```python
from build123d import *

# Parameters (mm, degrees)
FASE1_SIZE                           = 0.5
FASE2_SIZE                           = 1.3
SCHNITT_LINEAR_AUSTRAGEN1_DEPTH      = 15.75
SCHNITT_LINEAR_AUSTRAGEN1_DEPTH_BACK = 15.75
SKIZZE4_OUTSIDE_W                    = 40.932
SKIZZE4_OUTSIDE_H                    = 40.932
SKIZZE4_OUTSIDE_W_2                  = 20
SKIZZE4_OUTSIDE_H_2                  = 17
SCHNITT_LINEAR_AUSTRAGEN2_DEPTH      = 0.5


with BuildPart() as part:
    # Skizze2 → Rotation1 (revolve)
    with BuildSketch(Plane(origin=(0, 0, 0), x_dir=(0, 0, -1), z_dir=(1, 0, 0))):
        Polygon((0, 14.75), (-1.5, 14.75), (-1.5, 13), (-2, 13), (-2, 5.942548531), (-2.8, 5.942548531), (-2.8, 5), (-16.75, 5), (-16.75, 3.125), (-2.65, 3.125), (-2.65, 0.9), (5.25, 0.9), (5.25, 2.5), (0, 2.5), (0, 7.5), (0.5, 7.5), (0.5, 9.5), (0, 9.5), (0, 12.65), (-0.8, 12.65), (-0.8, 14.15), (0, 14.15), align=None)
    revolve(axis=Axis((0, 0, -10.606367747), (0, 0, 1)))

    # Fase1
    fase1_edges = [part.edges().sort_by_distance(p)[0] for p in [
        (0, -14.75, 1.5),
    ]]
    chamfer(fase1_edges, length=FASE1_SIZE)

    # Fase2
    fase2_edges = [part.edges().sort_by_distance(p)[0] for p in [
        (0, -3.125, 16.75),
    ]]
    chamfer(fase2_edges, length=FASE2_SIZE)

    # Skizze3 → Schnitt-Linear austragen1 (cut, two sides)
    with BuildSketch(Plane(origin=(0, 0, 0), x_dir=(1, 0, 0), z_dir=(0, 1, 0))) as schnitt_linear_austragen1_sk:
        with BuildLine():
            Line((1.85, -8.6), (1.85, -16.75))
            ThreePointArc((1.85, -16.75), (0, -18.6), (-1.85, -16.75))
            Line((-1.85, -16.75), (-1.85, -8.6))
            ThreePointArc((-1.85, -8.6), (0, -6.75), (1.85, -8.6))
        make_face()
    extrude(amount=SCHNITT_LINEAR_AUSTRAGEN1_DEPTH, mode=Mode.SUBTRACT)
    extrude(schnitt_linear_austragen1_sk.sketch, amount=-SCHNITT_LINEAR_AUSTRAGEN1_DEPTH_BACK, mode=Mode.SUBTRACT)

    # Skizze4 outside → Schnitt-Linear austragen2 (cut)
    with BuildSketch(Plane(origin=(0, 0, -0.5), x_dir=(-1, 0, 0), z_dir=(0, 0, -1))):
        Rectangle(SKIZZE4_OUTSIDE_W, SKIZZE4_OUTSIDE_H)
        Rectangle(SKIZZE4_OUTSIDE_W_2, SKIZZE4_OUTSIDE_H_2, mode=Mode.SUBTRACT)
    extrude(amount=-SCHNITT_LINEAR_AUSTRAGEN2_DEPTH, mode=Mode.SUBTRACT)


solid = part.part
```
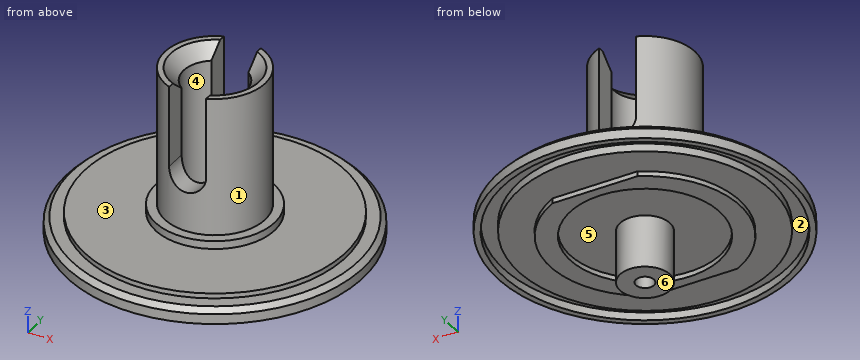
The model under review builds one solid part; all positions refer to its coordinate system, in mm. Face numbers are marked on the shaded views. A direction names the side the tool comes from. Coordinates: 2 decimals unless noted, no trailing zeros. Write each loop counter-clockwise with the first axis right and the second up, starting at its lowest first coordinate (ties: lowest second). Pieces come first, ordered by that corner, then holes.
1) The part is to be moulded in two halves that separate along Y. For the marked faces 1, 2 and 3, say which applies: pulls with the +Y half, pulls with the -Y half, needs draft (parallel to the pull), parting line crosses it, or undercut.
2) To check wall thickness, follow probe 1 along X at (y, z) = (0, 0.2); probe 2 along Y at (x, z) = (0, -0.1). State the ranges of each line that lie inside material, in increasing order.
3) Clearance check with flat-ended pins moving along their axes: pin 1 Ø1 at (x, y) = (9, 7.5) entering from +Z; pin 2 Ø2.5 at (y, z) = (4, 13) entering from +X; pin 3 Ø5 at (x, y) = (-1, -1) entering from +Z. State where each tip first meets the part, or that it passes through.
4) We need section A-A on z = 10.25. State the section outline as (x, y) points (3 decimals), then the cut area to 3 significant figures.
5) Machinability: for the marked faces 4, 5 and 6, which of the approach directions +Z, -Z, +X, -X, +Y, -Y give a long, thin tool a straight path to every point of the face, cutting with its end or side? Answer none if there is none.
6) We need section B-B on z = 4.5. State the section outline as (x, y) points (3 decimals), then the cut area to 3 significant figures.
Answer list:
1. face 1: parting line crosses it
1. face 2: undercut
1. face 3: needs draft
2. probe 1: x = -14.75 to -14.15, -12.65 to -0.9, 0.9 to 12.65, 14.15 to 14.75
2. probe 2: y = -8.5 to -7.5, -2.5 to -0.9, 0.9 to 2.5, 7.5 to 8.5
3. pin 1: stops at z = 2
3. pin 2: stops at x = 4.18
3. pin 3: stops at z = 16.24
4. outline: (-1.85, -4.645) - (-1.85, -2.519) arc R3.125 cw to (-1.85, 2.519) - (-1.85, 4.645) arc R5 ccw to start; (1.85, -4.645) arc R5 ccw to (1.85, 4.645) - (1.85, 2.519) arc R3.125 cw to (1.85, -2.519) - close
4. area: 33.4 mm2
5. face 4: +Z
5. face 5: -Z
5. face 6: -Z, +X, -X, +Y, -Y
6. outline: circle Ø10 at (0, 0); hole circle Ø6.25 at (0, 0)
6. area: 47.9 mm2
